from build123d import *

# Parameters (mm, degrees)
SALIENTE_EXTRUIR1_DEPTH = 23
CROQUIS1_4_R            = 9.5
SALIENTE_EXTRUIR2_DEPTH = 2
CROQUIS1_6_R            = 9.5
CROQUIS1_6_R_2          = 8.25
SALIENTE_EXTRUIR3_DEPTH = 4
CROQUIS2_W              = 12.2
CROQUIS2_H              = 4.7
CORTAR_EXTRUIR4_DEPTH   = 4
REDONDEO1_R             = 1
REDONDEO2_R             = 1


with BuildPart() as part:
    # Croquis1 → Saliente-Extruir1 (new body)
    with BuildSketch(Plane(origin=(0, 0, 0), x_dir=(1, 0, 0), z_dir=(0, 1, 0))):
        with BuildLine():
            Line((-34.110779311, 19.491025662), (16.889220689, 19.491025662))
            ThreePointArc((16.889220689, 19.491025662), (18.303434251, 18.905239224), (18.889220689, 17.491025662))
            Line((18.889220689, 17.491025662), (18.889220689, -19.008974338))
            ThreePointArc((18.889220689, -19.008974338), (18.303434251, -20.423187901), (16.889220689, -21.008974338))
            ThreePointArc((16.889220689, -21.008974338), (5.92906558, -25.54881923), (1.389220689, -36.508974338))
            ThreePointArc((1.389220689, -36.508974338), (0.803434251, -37.923187901), (-0.610779311, -38.508974338))
            Line((-0.610779311, -38.508974338), (-16.610779311, -38.508974338))
            ThreePointArc((-16.610779311, -38.508974338), (-18.024992874, -37.923187901), (-18.610779311, -36.508974338))
            ThreePointArc((-18.610779311, -36.508974338), (-23.150624203, -25.54881923), (-34.110779311, -21.008974338))
            ThreePointArc((-34.110779311, -21.008974338), (-35.524992874, -20.423187901), (-36.110779311, -19.008974338))
            Line((-36.110779311, -19.008974338), (-36.110779311, 17.491025662))
            ThreePointArc((-36.110779311, 17.491025662), (-35.524992874, 18.905239224), (-34.110779311, 19.491025662))
        make_face()
        with BuildLine():
            ThreePointArc((-32.110779311, 17.491025662), (-33.524992874, 16.905239224), (-34.110779311, 15.491025662))
            Line((-34.110779311, 15.491025662), (-34.110779311, -17.111809597))
            ThreePointArc((-34.110779311, -17.111809597), (-33.59574672, -18.451537851), (-32.315907517, -19.101262391))
            ThreePointArc((-32.315907517, -19.101262391), (-21.736410641, -24.134605668), (-16.703067364, -34.714102544))
            ThreePointArc((-16.703067364, -34.714102544), (-16.053342824, -35.993941747), (-14.71361457, -36.508974338))
            Line((-14.71361457, -36.508974338), (-2.507944053, -36.508974338))
            ThreePointArc((-2.507944053, -36.508974338), (-1.168215799, -35.993941747), (-0.518491259, -34.714102544))
            ThreePointArc((-0.518491259, -34.714102544), (4.514852018, -24.134605668), (15.094348894, -19.101262391))
            ThreePointArc((15.094348894, -19.101262391), (16.374188097, -18.451537851), (16.889220689, -17.111809597))
            Line((16.889220689, -17.111809597), (16.889220689, 15.491025662))
            ThreePointArc((16.889220689, 15.491025662), (16.303434251, 16.905239224), (14.889220689, 17.491025662))
            Line((14.889220689, 17.491025662), (-32.110779311, 17.491025662))
        make_face(mode=Mode.SUBTRACT)
    extrude(amount=SALIENTE_EXTRUIR1_DEPTH)

    # Croquis1_4 → Saliente-Extruir2 (add)
    with BuildSketch(Plane(origin=(0, 0, 0), x_dir=(1, 0, 0), z_dir=(0, 1, 0))):
        with BuildLine():
            Line((-32.110779311, 17.491025662), (14.889220689, 17.491025662))
            ThreePointArc((14.889220689, 17.491025662), (16.303434251, 16.905239224), (16.889220689, 15.491025662))
            Line((16.889220689, 15.491025662), (16.889220689, -17.111809597))
            ThreePointArc((16.889220689, -17.111809597), (16.374188097, -18.451537851), (15.094348894, -19.101262391))
            ThreePointArc((15.094348894, -19.101262391), (4.514852018, -24.134605668), (-0.518491259, -34.714102544))
            ThreePointArc((-0.518491259, -34.714102544), (-1.168215799, -35.993941747), (-2.507944053, -36.508974338))
            Line((-2.507944053, -36.508974338), (-14.71361457, -36.508974338))
            ThreePointArc((-14.71361457, -36.508974338), (-16.053342824, -35.993941747), (-16.703067364, -34.714102544))
            ThreePointArc((-16.703067364, -34.714102544), (-21.736410641, -24.134605668), (-32.315907517, -19.101262391))
            ThreePointArc((-32.315907517, -19.101262391), (-33.59574672, -18.451537851), (-34.110779311, -17.111809597))
            Line((-34.110779311, -17.111809597), (-34.110779311, 15.491025662))
            ThreePointArc((-34.110779311, 15.491025662), (-33.524992874, 16.905239224), (-32.110779311, 17.491025662))
        make_face()
        with Locations(Location((4.889220689, 0, 0), (0, 0, 270))):
            Circle(CROQUIS1_4_R, mode=Mode.SUBTRACT)
        with Locations(Location((-22.110779311, 0, 0), (0, 0, 270))):
            Circle(CROQUIS1_4_R, mode=Mode.SUBTRACT)
    extrude(amount=SALIENTE_EXTRUIR2_DEPTH)

    # Croquis1_6 → Saliente-Extruir3 (add)
    # profile 1 of 2: a face of its own
    with BuildSketch(Plane(origin=(0, 0, 0), x_dir=(1, 0, 0), z_dir=(0, 1, 0))):
        with Locations(Location((-22.110779311, 0, 0), (0, 0, 270))):
            Circle(CROQUIS1_6_R)
        with Locations(Location((-22.110779311, 0, 0), (0, 0, 270))):
            Circle(CROQUIS1_6_R_2, mode=Mode.SUBTRACT)
    # profile 2 of 2: a face of its own
    with BuildSketch(Plane(origin=(0, 0, 0), x_dir=(1, 0, 0), z_dir=(0, 1, 0))):
        with Locations(Location((4.889220689, 0, 0), (0, 0, 270))):
            Circle(CROQUIS1_6_R)
        with Locations(Location((4.889220689, 0, 0), (0, 0, 270))):
            Circle(CROQUIS1_6_R_2, mode=Mode.SUBTRACT)
    extrude(amount=SALIENTE_EXTRUIR3_DEPTH)

    # Croquis2 → Cortar-Extruir4 (cut)
    with BuildSketch(Plane.XY.offset(38.508974338)):
        with Locations((-8.713971977, 13.114927271)):
            Rectangle(CROQUIS2_W, CROQUIS2_H)
    extrude(amount=-CORTAR_EXTRUIR4_DEPTH, mode=Mode.SUBTRACT)

    # Redondeo1
    redondeo1_edges = [part.edges().sort_by_distance(p)[0] for p in [
        (-22.110779311, 2, -9.5),
    ]]
    fillet(redondeo1_edges, radius=REDONDEO1_R)

    # Redondeo2
    redondeo2_edges = [part.edges().sort_by_distance(p)[0] for p in [
        (4.889220689, 2, -9.5),
    ]]
    fillet(redondeo2_edges, radius=REDONDEO2_R)


solid = part.part
CAD build for the part. Positions are in the model's coordinates, mm. A direction names the side the tool comes from. Coordinates: 2 decimals unless noted, no trailing zeros. Loops run counter-clockwise (first coordinate to the right, second up) from the corner with the lowest first, then second, coordinate; pieces in that order, holes last. Notation, with made-up numbers: (-13, 22.5) - (43, 22.5) arc R30 ccw to (43, 60.5) - close; hole circle Ø7 at (-1.75, 38.5). An arc over 180 degrees is marked (long way). Write item = value, one per line. Start each with the question number.
Q1. Drill centre lines: L1, parallel to X at y = 3.05, z = 0; L2, parallel to X at y = 1.1, z = 0; L3, parallel to X at y = 12.5, z = -7. Where is each one in solid material? Low to high.
Q2. Flat gauge pins, fed straight in: pin 1 Ø1 at (x, z) = (-10.5, 38) entering from -Y; pin 2 Ø9.5 at (x, z) = (3, -4) entering from +Y; pin 3 Ø10 at (y, z) = (9.5, 31.5) entering from -X; pin 4 Ø0.6 at (y, z) = (14, 37) entering from -X. Where does each tip first touch, or does it go through?
Q3. Cut at B-B, the plane z = 0. List the corners of the cut face in (x, y).
Q4. Pull direction X, two halves, no side cores. Call faces 4 (the flat face through (18.889, 11, 1)), 5 (the cylindrical face through (-35.54, 11.34, -18.89)), 6 (the cylindrical face through (16.32, 12.35, -16.89)): pulls with the +X half, pulls with the -X half, needs draft (parallel to the pull), parting line crosses it, or undercut.
Q5. Which spindle directions (+Z, -Z, +X, -X, +Y, -Y) get a long thin tool onto all of the face, cutting with end or side? Do faces 1 (the flat face through (-9, 10, 36.509)), 2 (the flat face through (-9, 10.765, 38)), 3 (the cylindrical face through (0.819, 11.339, 37.908)). Say none if no direction does.
Q6. Cut at D-D, the plane z = 23.5. List the corners of the cut face in (x, y).
Q7. Cut at C-C, the plane y = 14. List the corners of the cut face in (x, z), then the cut area to 3 significant figures.
Q8. Cut at A-A, the plane y = 17.5. List the corners of the cut face in (x, z).
Computed:
q1.L1 = -36.11 to -34.11, -31.61 to -30.36, -13.86 to -12.61, -4.61 to -3.36, 13.14 to 14.39, 16.89 to 18.89
q1.L2 = -36.11 to -30.36, -13.86 to -3.36, 13.14 to 18.89
q1.L3 = -36.11 to -34.11, 16.89 to 18.89
q2.pin_1 = 0
q2.pin_2 = 4
q2.pin_3 = -22.28
q2.pin_4 = -18.6
q3.outline = (-36.11, 0) - (-30.36, 0) - (-30.36, 4) - (-31.61, 4) - (-31.61, 3) arc R1 cw to (-32.61, 2) - (-34.11, 2) - (-34.11, 23) - (-36.11, 23) - close; (-13.86, 0) - (-3.36, 0) - (-3.36, 4) - (-4.61, 4) - (-4.61, 3) arc R1 cw to (-5.61, 2) - (-11.61, 2) arc R1 cw to (-12.61, 3) - (-12.61, 4) - (-13.86, 4) - close; (13.14, 0) - (18.89, 0) - (18.89, 23) - (16.89, 23) - (16.89, 2) - (15.39, 2) arc R1 cw to (14.39, 3) - (14.39, 4) - (13.14, 4) - close
q4.face_4 = pulls with the +X half
q4.face_5 = pulls with the -X half
q4.face_6 = undercut
q5.face_1 = +Y
q5.face_2 = +Z
q5.face_3 = +Z, +X, +Y, -Y
q6.outline = (-25.68, 0) - (8.46, 0) - (8.46, 23) - (5.18, 23) - (5.18, 2) - (-22.41, 2) - (-22.41, 23) - (-25.68, 23) - close
q7.outline = (-36.11, -17.49) arc R2 ccw to (-34.11, -19.49) - (16.89, -19.49) arc R2 ccw to (18.89, -17.49) - (18.89, 19.01) arc R2 ccw to (16.89, 21.01) arc R15.5 cw to (1.39, 36.51) arc R2 ccw to (-0.61, 38.51) - (-2.61, 38.51) - (-2.61, 36.51) - (-2.51, 36.51) arc R2 cw to (-0.52, 34.71) arc R17.5 ccw to (15.09, 19.1) arc R2 cw to (16.89, 17.11) - (16.89, -15.49) arc R2 cw to (14.89, -17.49) - (-32.11, -17.49) arc R2 cw to (-34.11, -15.49) - (-34.11, 17.11) arc R2 cw to (-32.32, 19.1) arc R17.5 ccw to (-16.7, 34.71) arc R2 cw to (-14.81, 36.51) - (-14.81, 38.51) - (-16.61, 38.51) arc R2 ccw to (-18.61, 36.51) arc R15.5 cw to (-34.11, 21.01) arc R2 ccw to (-36.11, 19.01) - close
q7.area = 383 mm²
q8.outline = (-36.11, -17.49) arc R2 ccw to (-34.11, -19.49) - (16.89, -19.49) arc R2 ccw to (18.89, -17.49) - (18.89, 19.01) arc R2 ccw to (16.89, 21.01) arc R15.5 cw to (1.39, 36.51) arc R2 ccw to (-0.61, 38.51) - (-16.61, 38.51) arc R2 ccw to (-18.61, 36.51) arc R15.5 cw to (-34.11, 21.01) arc R2 ccw to (-36.11, 19.01) - close; hole (-34.11, -15.49) arc R2 ccw to (-32.11, -17.49) - (14.89, -17.49) arc R2 ccw to (16.89, -15.49) - (16.89, 17.11) arc R2 ccw to (15.09, 19.1) arc R17.5 cw to (-0.52, 34.71) arc R2 ccw to (-2.51, 36.51) - (-14.71, 36.51) arc R2 ccw to (-16.7, 34.71) arc R17.5 cw to (-32.32, 19.1) arc R2 ccw to (-34.11, 17.11) - close
